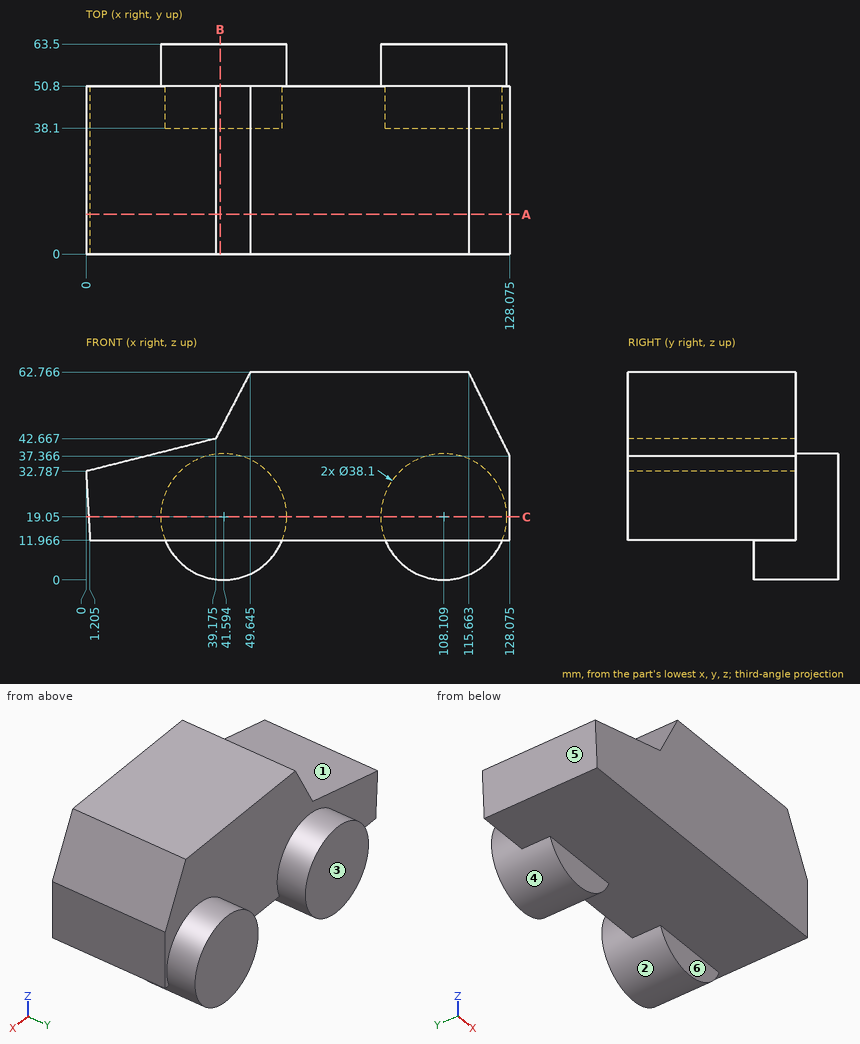
The figure shows three views and two pictorial views of one solid part (mm, origin at its lowest corner). Answer the questions. A direction names the side the tool comes from. Round coordinates to 2 decimals unless told otherwise and drop trailing zeros. Order: outer loops, then holes, each group sorted by start corner. A loop starts at its lowest first (then second) coordinate and runs counter-clockwise, first axis right, second up. Notation, with made-up numbers: M 70,84.25 L 107,84.25 A30 cw 107,121.25 Z; hole C -27,-11 d1. An arc over 180 degrees is marked long. Answer in a Markdown table with one row per item. Add a question column.
1) Determine the mould class of the marked faces 1, 2 and 3 for opening direction X: pulls with the +X half, pulls with the -X half, needs draft (parallel to the pull), parting line crosses it, or undercut.
2) The part is cut by section B-B on x = 40.5. Determine the outline of the cut face in (y, z) (1 decimal), plus the area to 3 significant figures.
3) The part is cut by section A-A on y = 12. Determine the outline of the cut face in (x, z) (1 decimal), plus the area to 3 significant figures.
4) The part is cut by section C-C on z = 19.05. Determine the outline of the cut face in (x, y) (1 decimal), plus the area to 3 significant figures.
5) Flat-ended cylindrical pins translate along their axes: pin 1 Ø2 at (y, z) = (21.5, 52) entering from -X (1 decimal); pin 2 Ø1.5 at (x, z) = (93.5, 54) entering from +Y; pin 3 Ø3 at (y, z) = (22.5, 27) entering from -X. Find the tip coordinate at first contact, or state that the pin passes through.
6) Consider line 1 along Z through (x, y) = (108, 56.5); line 2 along Z through (x, y) = (86, 21.5) (1 decimal); line 3 along Y through (x, z) = (108.5, 46). Determine where each line is inside the solid, lowest interval first. Write a range as from..to.
7) Which of the six approach directions +Z, -Z, +X, -X, +Y, -Y give full straight-line access (tool end or side, diameter ignored) to the marked faces 4, 5 and 6?
Findings below:
| question | item | result |
|---|---|---|
| 1 | face 1 | pulls with the -X half |
| 1 | face 2 | undercut |
| 1 | face 3 | needs draft |
| 2 | outline | M 0,12 L 38.1,12 L 38.1,0 L 63.5,0 L 63.5,38.1 L 50.8,38.1 L 50.8,45.2 L 0,45.2 Z |
| 2 | area | 2,320 mm² |
| 3 | outline | M 0,32.8 L 1.2,12 L 128.1,12 L 128.1,37.4 L 115.7,62.8 L 49.6,62.8 L 39.2,42.7 Z |
| 3 | area | 5,250 mm² |
| 4 | outline | M 0.8,0 L 128.1,0 L 128.1,50.8 L 127.2,50.8 L 127.2,63.5 L 89.1,63.5 L 89.1,50.8 L 60.6,50.8 L 60.6,63.5 L 22.5,63.5 L 22.5,50.8 L 0.8,50.8 Z |
| 4 | area | 7,430 mm² |
| 5 | pin 1 | stops at x = 43.5 |
| 5 | pin 2 | stops at y = 50.8 |
| 5 | pin 3 | stops at x = 0.25 |
| 6 | line 1 | z = 0..38.1 |
| 6 | line 2 | z = 12..62.8 |
| 6 | line 3 | y = 0..50.8 |
| 7 | face 4 | +Y |
| 7 | face 5 | -Z, -X, +Y, -Y |
| 7 | face 6 | -Z, +X, -X, -Y |
